The model under review builds one solid part; all positions refer to its coordinate system, in mm. Face numbers are marked on the shaded views. A direction names the side the tool comes from. Coordinates: 2 decimals unless noted, no trailing zeros. Write each loop counter-clockwise with the first axis right and the second up, starting at its lowest first coordinate (ties: lowest second). Pieces come first, ordered by that corner, then holes.
1) Add section A-A, the plane y = 108.5. State the section outline as (x, z) points.
2) Add section D-D, the plane x = 7.25. State the section outline as (y, z) points.
3) For line 1 (Z direction, x = 0, y = 4.8); line 2 (Z direction, x = -4.5, y = 45); line 3 (X direction, y = 65.5, z = 6), list the stretches that pass through material, from the lowest coordinate up.
4) Add section C-C, the plane x = -0.5. Give the number of separate pieces and of enclosed holes in the cut face, then the cut area to 3 significant figures.
5) For P1, Ø3.5, axis at x = 0.5, y = 58.5, coming from the +Z side; P2, Ø6, axis at x = -1.5, z = 8, coming from the +Y side; P3, Ø8, axis at y = 62, z = 17.5, coming from the +X side; P4, Ø3, axis at x = 1, y = 60, coming from the -Z side, all flat-tipped, find the tip position at first contact; note any pin that passes through.
6) Machinability: for the marked faces 1, 2, 3 and 4, which of the approach directions +Z, -Z, +X, -X, +Y, -Y give a long, thin tool a straight path to every point of the face, cutting with its end or side? Answer none if there is none.
7) Mouldability with a two-part tool opening along X and no side actions: class the marked faces 5, 6 and 7 as released by +X, released by -X, zero draft, split by the parting line, or undercut.
8) Add section B-B, the plane z = -6.5. State the section outline as (x, y) points.
Autodesk Inventor part; units mm, degrees
ref_plane "YZ Plane" through (0, 0, 0) normal (1, 0, 0) x (0, 1, 0)
ref_plane "XZ Plane" through (0, 0, 0) normal (0, 1, 0) x (-1, 0, 0)
ref_plane "XY Plane" through (0, 0, 0) normal (0, 0, 1) x (1, 0, 0)
sketch "Sketch2" plane through (0, 0, 0) normal (0, 1, 0) x (-1, 0, 0)
  line L0 (5, 8.5) -> (-5, 8.5)
  line L1 (-5, 8.5) -> (-5, -8.5)
  line L2 (-5, -8.5) -> (5, -8.5)
  line L3 (5, -8.5) -> (5, 8.5)
  line L4 (5, 8.5) -> (-5, -8.5) construction
  line L5 (-5, 8.5) -> (5, -8.5) construction
  line L6 (9, 12.5) -> (-9, 12.5)
  line L7 (-9, 12.5) -> (-9, -12.5)
  line L8 (-9, -12.5) -> (9, -12.5)
  line L9 (9, -12.5) -> (9, 12.5)
  point P0 (0, 0)
  dimension "d0" = 17
  dimension "d1" = 10
  dimension "d2" = 4
extrude "Extrusion1" add sketch "Sketch2" along normal blind 130
sketch "Sketch3" plane through (9, 0, -12.5) normal (0, 0, -1) x (-1, 0, 0)
  line L0 (0, 0) -> (0, 130)
  line L1 (18, 0) -> (18, 130)
  line L2 (0, 0) -> (18, 0)
  line L3 (18, 0) -> (18, 6)
  line L4 (18, 6) -> (0, 6)
  line L5 (0, 6) -> (0, 0)
  point P0 (9, 0)
  point P1 (0, 6)
  dimension "d5" = 6
extrude "Extrusion2" add sketch "Sketch3" along normal blind 10
sketch "Sketch4" plane through (-9, 6, -12.5) normal (0, 1, 0) x (1, 0, 0)
  circle A0 centre (9, 5) radius 3.25
  circle A1 centre (9, 5) radius 1.7
  line L0 (0, 0) -> (0, 10)
  line L1 (0, 10) -> (18, 10)
  point P0 (9, -12.5)
  point P1 (0, 5)
  point P2 (9, 10)
  dimension "d8" = 6.5
  dimension "d9" = 3.4
extrude "Extrusion3" cut sketch "Sketch4" against normal blind 10 contours A1
extrude "Extrusion4" cut sketch "Sketch4" against normal blind 3
sketch "Sketch5" plane through (9, 0, 12.5) normal (1, 0, 0) x (0, 0, -1)
  line L0 (0, 0) -> (0, 130)
  line L1 (0, 130) -> (0, 132.1872)
  line L2 (25, 130) -> (0, 130)
  line L3 (0, 132.1872) -> (25, 130)
  line L4 (0, 132.1872) -> (-9.9619, 133.0588)
  line L5 (-9.9619, 133.0588) -> (-10.1519, 130.8882)
  line L6 (-10.1519, 130.8882) -> (0, 130)
  line L7 (25, 6) -> (25, 130)
  point P0 (12.5, 0)
  dimension "d14" = 5
  dimension "d18" = 10
extrude "Extrusion5" add sketch "Sketch5" against normal up to surface (18 mm away)
extrude "Extrusion6" cut sketch "Sketch2" along normal through all contours L3 L2 L1 L0
sketch "Sketch6" plane through (-9, 130, 12.5) normal (0, -0.9961947, 0.0871557) x (1, 0, 0)
  circle A0 centre (9, 5.0953) radius 2.75
  circle A1 centre (9, 5.0953) radius 1.7
  line L0 (0, 10.1906) -> (0, 0)
  line L1 (18, 10.1906) -> (0, 10.1906)
  point P0 (9, -23.7827)
  point P1 (0, 5.0953)
  point P2 (9, 10.1906)
  dimension "d23" = 5.5
  dimension "d24" = 3.4
extrude "Extrusion7" cut sketch "Sketch6" against normal blind 10 contours A1
extrude "Extrusion8" cut sketch "Sketch6" against normal blind 2
mirror "Mirror1" about plane through (0, 0, 0) normal (0, 0, 1) of "Extrusion2", "Extrusion3", "Extrusion4"
fillet "Fillet1" radius 3 6 edges at (9, 68, -12.5) (-9, 68, -12.5) (9, 68, 12.5) (-9, 68, 12.5) (9, 131.9735, 22.5569) (-9, 131.9735, 22.5569)
properties part number "Path Holder"
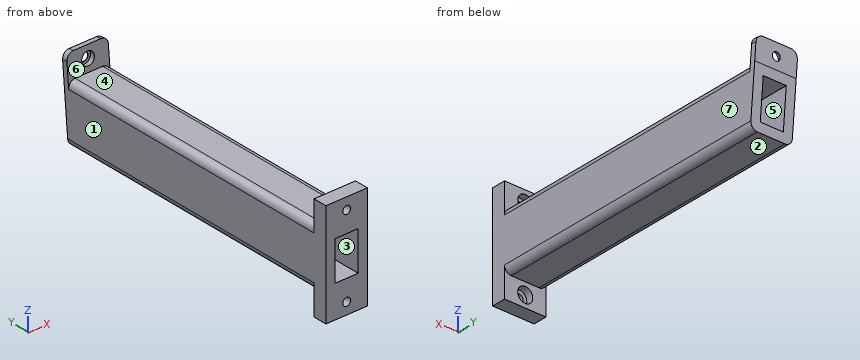
Geometry results:
1. outline: (-9, -9.5) arc R3 ccw to (-6, -12.5) - (6, -12.5) arc R3 ccw to (9, -9.5) - (9, 9.5) arc R3 ccw to (6, 12.5) - (-6, 12.5) arc R3 ccw to (-9, 9.5) - close; hole (-5, -8.5) - (5, -8.5) - (5, 8.5) - (-5, 8.5) - close
2. outline: (0, -22.5) - (6, -22.5) - (6, -12.23) - (130.02, -12.23) - (132.19, 12.5) - (133.04, 22.19) - (130.86, 22.38) - (129.98, 12.23) - (6, 12.23) - (6, 22.5) - (0, 22.5) - close
3. line 1: z = -22.5 to -20.75, -14.25 to -8.5, 8.5 to 14.25, 20.75 to 22.5
3. line 2: z = -12.5 to -8.5, 8.5 to 12.5
3. line 3: x = -9 to -5, 5 to 9
4. separate pieces: 5
4. enclosed holes: 0
4. area: 1,120 mm2
5. P1: stops at z = 12.5
5. P2: stops at y = 132.06
5. P3: passes through
5. P4: stops at z = -12.5
6. face 1: +Z, -Z, -X, +Y, -Y
6. face 2: -Z, +X, -X, +Y
6. face 3: +Y, -Y
6. face 4: +Z, +X, -X
7. face 5: undercut
7. face 6: zero draft
7. face 7: released by +X
8. outline: (-9, 0) - (-5, 0) - (-5, 130.52) - (-9, 130.52) - close; (5, 0) - (9, 0) - (9, 130.52) - (5, 130.52) - close
